For this review, take the finished solid that the model builds, in its own axes (mm). Coordinates: 2 decimals unless noted, no trailing zeros.
```python
from build123d import *

# Parameters (mm, degrees)
SKETCH2_R          = 7.75
SKETCH2_R_2        = 7.9375
SKETCH2_R_3        = 9
CUT_EXTRUDE1_DEPTH = 85.463711951


with BuildPart() as part:
    # Sketch1 → Revolve1 (revolve)
    with BuildSketch(Plane(origin=(0, 0, 0), x_dir=(0, 0, -1), z_dir=(1, 0, 0)), mode=Mode.PRIVATE) as revolve1_sk:
        with BuildLine():
            Line((0, 0), (0, 52.809927725))
            ThreePointArc((0, 52.809927725), (0.130798304, 53.244522907), (0.479738309, 53.534733247))
            Line((0.479738309, 53.534733247), (0.872854821, 53.701601306))
            ThreePointArc((0.872854821, 53.701601306), (1.6002, 54.8005), (0.872854821, 55.899398694))
            Line((0.872854821, 55.899398694), (0.479738309, 56.066266753))
            ThreePointArc((0.479738309, 56.066266753), (0.130798304, 56.356477093), (0, 56.791072275))
            Line((0, 56.791072275), (0, 59.4614))
            Line((0, 59.4614), (2.8448, 59.4614))
            Line((2.8448, 59.4614), (7.9248, 45.504214709))
            Line((7.9248, 45.504214709), (7.9248, 0))
            Line((7.9248, 0), (0, 0))
        make_face()
    revolve(revolve1_sk.sketch.rotate(Axis((0, 0, 0), (0, 0, -1)), 90), axis=Axis((0, 0, 0), (0, 0, -1)))

    # Sketch2 → Cut-Extrude1 (cut, through all)
    with BuildSketch(Plane(origin=(0, 0, -7.9248), x_dir=(-1, 0, 0), z_dir=(0, 0, -1))):
        with Locations((-23.121403313, 22.329574432)):
            Circle(SKETCH2_R)
        with Locations((23.014902328, 22.329574432)):
            Circle(SKETCH2_R)
        with Locations((0, 31.198057894)):
            Circle(SKETCH2_R_2)
        Circle(SKETCH2_R_2)
        with Locations((-28.2480994, -8.614227209)):
            Circle(SKETCH2_R_2)
        with Locations((0, -32.377727799)):
            Circle(SKETCH2_R_3)
        with Locations((28.850997909, -8.614227209)):
            Circle(SKETCH2_R_2)
    extrude(amount=-CUT_EXTRUDE1_DEPTH, mode=Mode.SUBTRACT)


solid = part.part
```
Q1. Consider section A-A (x = 0). Count the separate pieces of the cut face and the enclosed holes in it, then the cut area to 3 significant figures.
Q2. Wall thickness on probe 1 along X at (y, z) = (16, -1); probe 2 along Y at (x, z) = (-49, -0.5); probe 3 along Y at (x, z) = (9.5, -0.25): over which ranges is each line inside the solid? List them lowest first.
Q3. For pin 1 Ø4 at (y, z) = (-28, -3) entering from +X; pin 2 Ø1.5 at (x, z) = (-32, -1.5) entering from +Y, all flat-tipped, find the tip position at first contact; note any pin that passes through.
Q4. The part is to be moulded in two halves that separate along Y. For faces 1 (the face through (1.72, -7.75, -4.02)), 2 (the face through (1, 11, 0)), 3 (the face through (56.716, -17.861, -1.442)), say which applies: +Y half, -Y half, draft (parallel to the pull), parting line (faces both ways), or undercut.
Model answer:
1. separate pieces: 4
1. enclosed holes: 0
1. area: 470 mm2
2. probe 1: x = -57.27 to -53.49, -51.33 to -27.49, -18.54 to 18.65, 27.59 to 51.33, 53.49 to 57.27
2. probe 2: y = -33.68 to -27.23, -21.58 to 21.58, 27.23 to 33.68
2. probe 3: y = -58.7 to -55.41, -52.53 to 52.53, 55.41 to 58.7
3. pin 1: stops at x = 53.47
3. pin 2: stops at y = 50.59
4. face 1: undercut
4. face 2: draft
4. face 3: parting line
